Answer from the drawing. Dimensions are ordinates in mm from the lowest x, y and z of the part. A direction names the side the tool comes from. Round coordinates to 2 decimals unless told otherwise and drop trailing zeros. Write each loop counter-clockwise with the first axis right and the second up, starting at its lowest first coordinate (ties: lowest second). Pieces come first, ordered by that corner, then holes. Notation, with made-up numbers: (70.5, 81) - (123.5, 81) arc R35 ccw to (123.5, 115) - close; hole circle Ø3 at (-23, -21.5). An arc over 180 degrees is marked (long way). Answer as CSV lines item,"result". Start each with the question number.
1) Find section B-B on y = 10. Determine the outline of the cut face in (x, z), then the cut area to 3 significant figures.
2) Consider line 1 along Z through (x, y) = (36, 18.25); line 2 along Z through (x, y) = (37.85, 4); line 3 along Z through (x, y) = (17.5, 5). Determine where each line is inside the solid, lowest interval first.
3) Find section A-A on x = 37.85. Determine the outline of the cut face in (y, z).
4) Each of these flat-tipped pins is pushed along its axis until it touches: pin 1 (4 mm diameter, centred on y = 2.5, z = 23.5, fed in from +X); pin 2 (7 mm diameter, centred on x = 37.85, z = 6, fed in from +Y); pin 3 (8 mm diameter, centred on y = 17.5, z = 16, fed in from +X) (1 decimal); pin 4 (4.5 mm diameter, centred on y = 10, z = 22.7, fed in from +X). Where does it stop, or does it pass through?
5) Find section D-D on z = 38. Determine the outline of the cut face in (x, y).
6) For a pull along Z with two mould halves and no side action, classify the marked faces 1, 2 and 3 as +Z half, -Z half, draft (parallel to the pull), parting line (faces both ways), or undercut.
7) Find section C-C on x = 26.5. Determine the outline of the cut face in (y, z), then the cut area to 3 significant figures.
8) Which of the six approach directions +Z, -Z, +X, -X, +Y, -Y give full straight-line access (tool end or side, diameter ignored) to the marked faces 4 and 5?
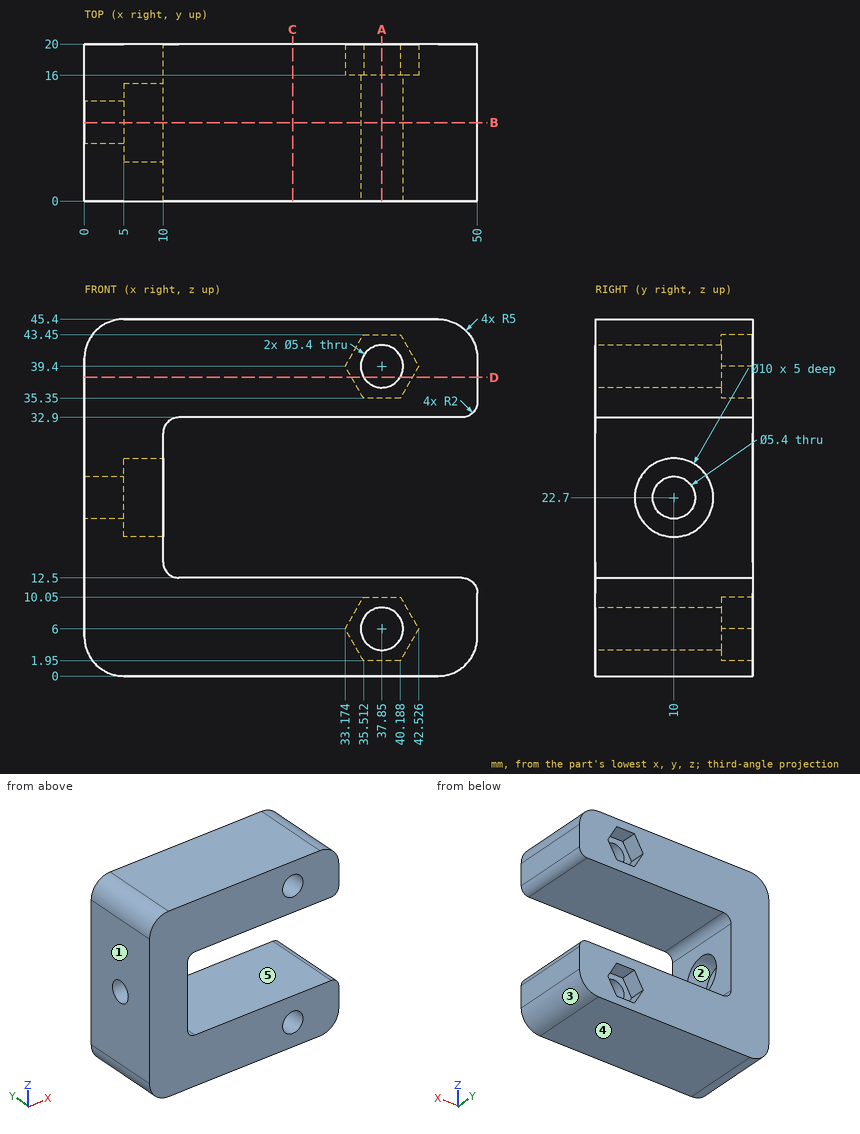
Check values:
1,outline,"(0, 5) arc R5 ccw to (5, 0) - (45, 0) arc R5 ccw to (50, 5) - (50, 10.5) arc R2 ccw to (48, 12.5) - (12, 12.5) arc R2 cw to (10, 14.5) - (10, 17.7) - (5, 17.7) - (5, 20) - (0, 20) - close; (0, 25.4) - (5, 25.4) - (5, 27.7) - (10, 27.7) - (10, 30.9) arc R2 cw to (12, 32.9) - (48, 32.9) arc R2 ccw to (50, 34.9) - (50, 40.4) arc R5 ccw to (45, 45.4) - (5, 45.4) arc R5 ccw to (0, 40.4) - close; hole circle Ø5.4 at (37.85, 6); hole circle Ø5.4 at (37.85, 39.4)"
1,area,"1,310 mm^2"
2,line 1,"z = 0 to 1.95, 10.05 to 12.5, 32.9 to 35.35, 43.45 to 45.4"
2,line 2,"z = 0 to 3.3, 8.7 to 12.5, 32.9 to 36.7, 42.1 to 45.4"
2,line 3,"z = 0 to 12.5, 32.9 to 45.4"
3,outline,"(0, 0) - (20, 0) - (20, 1.95) - (16, 1.95) - (16, 3.3) - (0, 3.3) - close; (0, 8.7) - (16, 8.7) - (16, 10.05) - (20, 10.05) - (20, 12.5) - (0, 12.5) - close; (0, 32.9) - (20, 32.9) - (20, 35.35) - (16, 35.35) - (16, 36.7) - (0, 36.7) - close; (0, 42.1) - (16, 42.1) - (16, 43.45) - (20, 43.45) - (20, 45.4) - (0, 45.4) - close"
4,pin 1,"stops at x = 10"
4,pin 2,"stops at y = 16"
4,pin 3,"stops at x = 49.3"
4,pin 4,"passes through"
5,outline,"(0, 0) - (35.54, 0) - (35.54, 16) - (33.98, 16) - (33.98, 20) - (0, 20) - close; (40.16, 0) - (50, 0) - (50, 20) - (41.72, 20) - (41.72, 16) - (40.16, 16) - close"
6,face 1,"draft"
6,face 2,"undercut"
6,face 3,"-Z half"
7,outline,"(0, 0) - (20, 0) - (20, 12.5) - (0, 12.5) - close; (0, 32.9) - (20, 32.9) - (20, 45.4) - (0, 45.4) - close"
7,area,"500 mm^2"
8,face 4,"-Z, +X, -X, +Y, -Y"
8,face 5,"+X, +Y, -Y"
